```python
from build123d import *

# Parameters (mm, degrees)
BOSS_EXTRUDE1_DEPTH = 342.9
CUT_EXTRUDE1_REACH  = 346.776
SKETCH2_R           = 4.7625


with BuildPart() as part:
    # Sketch1 → Boss-Extrude1 (new body)
    with BuildSketch(Plane(origin=(0, 0, 0), x_dir=(1, 0, 0), z_dir=(0, 1, 0))):
        Polygon((0, 0), (3.302, 0), (3.302, 22.098), (25.4, 22.098), (25.4, 25.4), (0, 25.4), align=None)
    extrude(amount=BOSS_EXTRUDE1_DEPTH)

    # Sketch2 → Cut-Extrude1 (cut, up to next)
    with BuildSketch(Plane(origin=(0, 0, -25.4), x_dir=(-1, 0, 0), z_dir=(0, 0, -1)), mode=Mode.PRIVATE) as cut_extrude1_sk1:
        with Locations((-12.7, 171.45)):
            Circle(SKETCH2_R)
    cut_extrude1_tool1 = extrude(cut_extrude1_sk1.sketch, amount=-CUT_EXTRUDE1_REACH, mode=Mode.PRIVATE) & part.part
    add(cut_extrude1_tool1.solids().sort_by_distance((12.7, 171.45, -25.4))[0], mode=Mode.SUBTRACT)


solid = part.part
```
Build history of the part. All positions in model axes, mm. A direction names the side the tool comes from. Round coordinates to 2 decimals unless told otherwise and drop trailing zeros. Loops run counter-clockwise (first coordinate to the right, second up) from the corner with the lowest first, then second, coordinate; pieces in that order, holes last.
Item 1: Saw through at B-B (x = 12.7). List the corners of the cut face in (y, z), then the cut area to 3 significant figures.
Item 2: Which spindle directions (+Z, -Z, +X, -X, +Y, -Y) get a long thin tool onto all of the face, cutting with end or side? Do faces 1 (the face through (3.302, 169, -11)), 2 (the face through (0, 169, -13)). Say none if no direction does.
Item 3: Two-plate mould, pull along Y, no slides. Class faces 3 (the face through (19, 169, -22.098)), 4 (the face through (3, 0, -18)), 5 (the face through (3, 342.9, -18)), 6 (the face through (13.32, 176.17, -23.77)): released by +Y, released by -Y, zero draft, split by the parting line, or undercut.
Item 4: Saw through at A-A (y = 171.45). List the corners of the cut face in (x, z).
Item 5: Drill centre lines: line 1 along Y through (x, z) = (12.7, -23.45); line 2 along Z through (x, y) = (22.5, 101.5); line 3 along X through (y, z) = (160, -13.5). Where is each one in solid material? Low to high.
Item 6: Pin check, flat tips, straight feed: P1, Ø6, axis at x = 10, y = 303, coming from the +Z side; P2, Ø11, axis at y = 216.5, z = -8.5, coming from the +X side; P3, Ø4, axis at x = 12.5, z = -21.5, coming from the +Y side; P4, Ø5.5, axis at x = 12.7, y = 171.45, coming from the -Z side. Stop position of each tip, or through.
Item 7: Saw through at D-D (z = -4). List the corners of the cut face in (x, y).
Item 8: Saw through at C-C (y = 77.5). List the corners of the cut face in (x, z), then the cut area to 3 significant figures.
Worked answers:
1. outline: (0, -25.4) - (166.69, -25.4) - (166.69, -22.1) - (0, -22.1) - close; (176.21, -25.4) - (342.9, -25.4) - (342.9, -22.1) - (176.21, -22.1) - close
1. area: 1,100 mm2
2. face 1: +Z, +X, +Y, -Y
2. face 2: +Z, -Z, -X, +Y, -Y
3. face 3: zero draft
3. face 4: released by -Y
3. face 5: released by +Y
3. face 6: undercut
4. outline: (0, -25.4) - (7.94, -25.4) - (7.94, -22.1) - (3.3, -22.1) - (3.3, 0) - (0, 0) - close; (17.46, -25.4) - (25.4, -25.4) - (25.4, -22.1) - (17.46, -22.1) - close
5. line 1: y = 0 to 166.69, 176.21 to 342.9
5. line 2: z = -25.4 to -22.1
5. line 3: x = 0 to 3.3
6. P1: stops at z = -22.1
6. P2: stops at x = 3.3
6. P3: stops at y = 342.9
6. P4: passes through
7. outline: (0, 0) - (3.3, 0) - (3.3, 342.9) - (0, 342.9) - close
8. outline: (0, -25.4) - (25.4, -25.4) - (25.4, -22.1) - (3.3, -22.1) - (3.3, 0) - (0, 0) - close
8. area: 157 mm2
